Check sheet for the modelled part. Datum: model origin and axes. Units: mm. Round coordinates to 2 decimals unless told otherwise and drop trailing zeros. Loops run counter-clockwise (first coordinate to the right, second up) from the corner with the lowest first, then second, coordinate; pieces in that order, holes last. Notation, with made-up numbers: (1, 89) -> (55, 89) arc R26 ccw to (55, 115) -> close; hole circle Ø4 at (32, -20). An arc over 180 degrees is marked (long way). Return JSON: item names as keys, results as strings.
from build123d import *

# Parameters (mm, degrees)
F0_R     = 57.15
F0_R_2   = 47.625
F1_DEPTH = 304.8
F2_R     = 6.35
F3_DEPTH = 57.151
F4_DEPTH = 57.151


with BuildPart() as f1:
    # F0 (on Top) → F1 (new body)
    with BuildSketch(Plane.XY):
        Circle(F0_R)
        Circle(F0_R_2, mode=Mode.SUBTRACT)
    extrude(amount=F1_DEPTH)

    # F2 (on Front) → F3 (cut, through all)
    with BuildSketch(Plane.XZ):
        with Locations((0, 82.55)):
            Circle(F2_R)
        with Locations((0, 158.75)):
            Circle(F2_R)
        with Locations((0, 234.95)):
            Circle(F2_R)
    extrude(amount=-F3_DEPTH, mode=Mode.SUBTRACT)

    # F2 (on Front) → F4 (cut, through all)
    with BuildSketch(Plane.XZ):
        with Locations((0, 82.55)):
            Circle(F2_R)
        with Locations((0, 158.75)):
            Circle(F2_R)
        with Locations((0, 234.95)):
            Circle(F2_R)
    extrude(amount=F4_DEPTH, mode=Mode.SUBTRACT)


solid = f1.part
Q1. Section check A-A (y = 0). Record the boundary of the cut face in (x, z) (3 decimals).
Results list:
{"outline": "(-57.15, 0) -> (-47.625, 0) -> (-47.625, 304.8) -> (-57.15, 304.8) -> close; (47.625, 0) -> (57.15, 0) -> (57.15, 304.8) -> (47.625, 304.8) -> close"}
Q2. Draft check along Z on faces 1 (the flat face through (-21, 43, 0)), 2 (the flat face through (-21, 43, 304.8)), 3 (the cylindrical face through (-0.827, -52.109, 165.046)), 4 (the cylindrical face through (-10.324, -46.492, 150.266)). Enter one of: released by +Z, released by -Z, zero draft, split by the parting line, or undercut.
Results list:
{"face 1": "released by -Z", "face 2": "released by +Z", "face 3": "undercut", "face 4": "zero draft"}
Q3. Go/stop test with flat-tipped pins: pin 1 (16.5 mm diameter, centred on x = 0, z = 158.75, fed in from -Y); pin 2 (3 mm diameter, centred on x = 14.5, z = 237.5, fed in from -Y); pin 3 (4 mm diameter, centred on y = 20.5, z = 84.5, fed in from -X); pin 4 (1.5 mm diameter, centred on x = -21, z = 42, fed in from +Y). Record where each tip stops, or that it passes through.
Results list:
{"pin 1": "y = -57.15", "pin 2": "y = -55.65", "pin 3": "x = -54.07", "pin 4": "y = 53.44"}
Q4. Section check C-C (x = -18). Record the boundary of the cut face in (y, z).
Results list:
{"outline": "(-54.24, 0) -> (-44.09, 0) -> (-44.09, 304.8) -> (-54.24, 304.8) -> close; (44.09, 0) -> (54.24, 0) -> (54.24, 304.8) -> (44.09, 304.8) -> close"}
Q5. Section check B-B (x = 0). Count the separate pieces of the cut face and the enclosed holes in it, then the cut area to 3 significant figures.
Results list:
{"separate pieces": "8", "enclosed holes": "0", "area": "5,080 mm^2"}
Q6. Material ranges on line 1 (Z direction, x = 0, y = -52.75); line 2 (Y direction, x = 0, z = 221.5) (3 decimals); line 3 (Y direction, x = 25.5, z = 267), recorded low to high.
Results list:
{"line 1": "0 to 76.2, 88.9 to 152.4, 165.1 to 228.6, 241.3 to 304.8", "line 2": "-57.15 to -47.625, 47.625 to 57.15", "line 3": "-51.15 to -40.22, 40.22 to 51.15"}
Q7. Section check D-D (z = 178). Record the boundary of the cut face in (x, y) (3 decimals).
Results list:
{"outline": "circle Ø114.3 at (0, 0); hole circle Ø95.25 at (0, 0)"}
